Could you check a few things on this drawing? It's one solid part, dimensions in mm from its lowest x, y, z. A direction names the side the tool comes from. Coordinates: 2 decimals unless noted, no trailing zeros. Loops run counter-clockwise (first coordinate to the right, second up) from the corner with the lowest first, then second, coordinate; pieces in that order, holes last. Notation, with made-up numbers: M -9,-8 L 2,-8 A24 ccw 2,15 Z; hole C 30,61.25 d10. An arc over 180 degrees is marked long. Answer as a JSON object with one key per item and string values. Group by question number.
Item 1: If I drill on line 1 (Z direction, x = 39, y = 7.5); line 2 (X direction, y = 10.5, z = 36.5); line 3 (Y direction, x = 39, z = 60), over which ranges is the centre line in solid material (lowest first)?
Item 2: Suppose I cut it at A-A (x = 43). Write out the boundary of the cut face in (y, z), then the cut area to 3 significant figures.
Item 3: Suppose I cut it at D-D (z = 10). Write out the boundary of the cut face in (x, y), then the cut area to 3 significant figures.
Item 4: We'd pull the mould along Z, two halves only. Please class the marked faces 4, 5 and 6: +Z half, -Z half, draft (parallel to the pull), parting line (faces both ways), or undercut.
Item 5: Which directions (+Z, -Z, +X, -X, +Y, -Y) give clear straight access to the entire face, cutting with the end or side of a thin tool? Please do the marked faces 1, 2 and 3.
Item 6: Suppose I cut it at C-C (x = 13.5). Write out the boundary of the cut face in (y, z).
Item 7: I'm going to push flat-ended pins straight in: pin 1 Ø1.5 at (y, z) = (22, 9.5) entering from +X; pin 2 Ø6 at (y, z) = (7, 38.5) entering from +X; pin 3 Ø1 at (y, z) = (8.5, 33) entering from -X; pin 4 Ø3 at (x, z) = (36, 13.5) entering from +Y. Where does each tip first touch, or does it pass through?
Item 8: Suppose I cut it at B-B (y = 6). Write out the boundary of the cut face in (x, z), then the cut area to 3 significant figures.
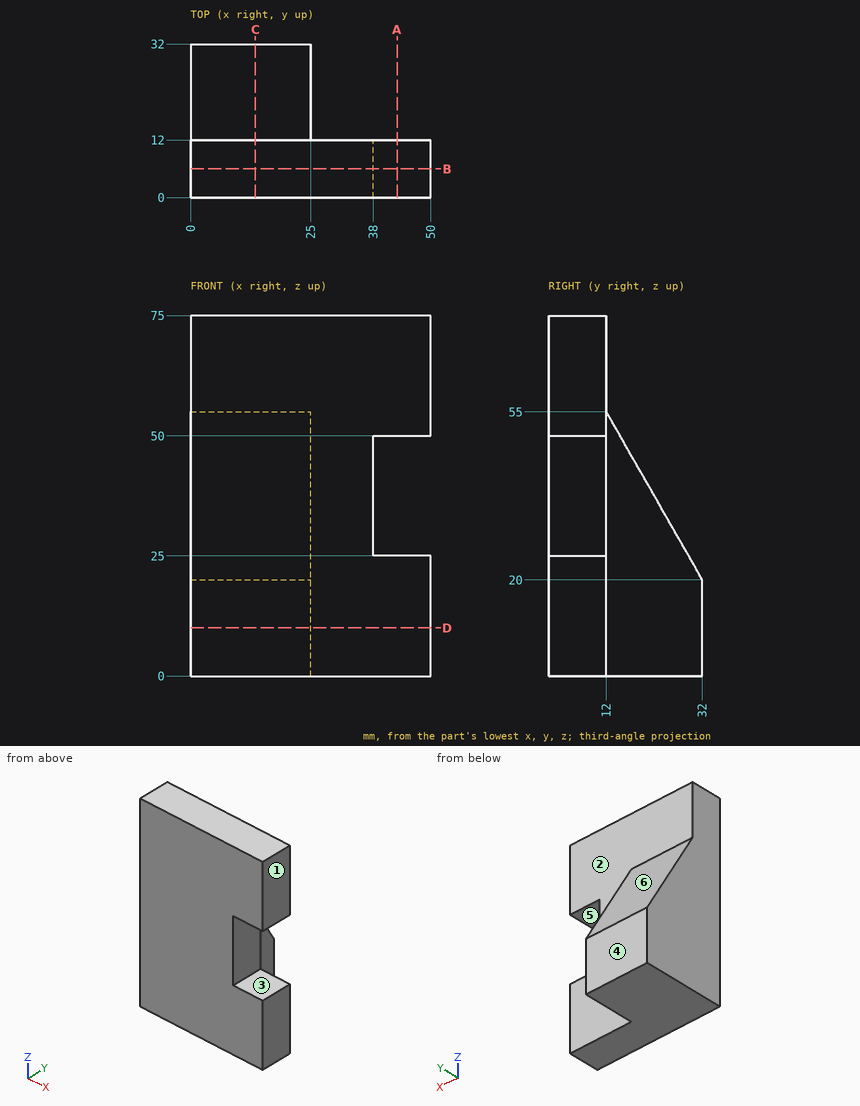
From the geometry:
{
 "1": {"line 1": "0 to 25, 50 to 75", "line 2": "0 to 38", "line 3": "0 to 12"},
 "2": {"outline": "M 0,0 L 12,0 L 12,25 L 0,25 Z; M 0,50 L 12,50 L 12,75 L 0,75 Z", "area": "600 mm2"},
 "3": {"outline": "M 0,0 L 50,0 L 50,12 L 25,12 L 25,32 L 0,32 Z", "area": "1,100 mm2"},
 "4": {"face 4": "draft", "face 5": "undercut", "face 6": "+Z half"},
 "5": {"face 1": "+Z, -Z, +X, +Y, -Y", "face 2": "+Z, +X, +Y", "face 3": "+X, +Y, -Y"},
 "6": {"outline": "M 0,0 L 32,0 L 32,20 L 12,55 L 12,75 L 0,75 Z"},
 "7": {"pin 1": "x = 25", "pin 2": "x = 38", "pin 3": "x = 0", "pin 4": "y = 12"},
 "8": {"outline": "M 0,0 L 50,0 L 50,25 L 38,25 L 38,50 L 50,50 L 50,75 L 0,75 Z", "area": "3,450 mm2"}
}
